```python
from build123d import *

# Parameters (mm, degrees)
BOSS_EXTRUDE1_DEPTH = 43.5102
CUT_EXTRUDE1_DEPTH  = 43.5102


with BuildPart() as part:
    # Sketch2 → Boss-Extrude1 (new body)
    with BuildSketch(Plane.XY):
        with BuildLine():
            Line((-4.366026501, 25.941944541), (-1.27, 34.448207442))
            ThreePointArc((-1.27, 34.448207442), (0, 34.47161), (1.27, 34.448207442))
            Line((1.27, 34.448207442), (4.366026501, 25.941944541))
            ThreePointArc((4.366026501, 25.941944541), (4.83385814, 25.858857079), (5.300112805, 25.767333549))
            Line((5.300112805, 25.767333549), (11.259888122, 32.580773709))
            ThreePointArc((11.259888122, 32.580773709), (12.452581833, 32.143819028), (13.628367585, 31.663219877))
            Line((13.628367585, 31.663219877), (13.442509735, 22.612952173))
            ThreePointArc((13.442509735, 22.612952173), (13.848735094, 22.366475142), (14.250442508, 22.11270138))
            Line((14.250442508, 22.11270138), (22.26906596, 26.31312595))
            ThreePointArc((22.26906596, 26.31312595), (23.223373486, 25.474827181), (24.14614861, 24.601939015))
            Line((24.14614861, 24.601939015), (20.703507542, 16.229955312))
            ThreePointArc((20.703507542, 16.229955312), (20.993263634, 15.8533768), (21.276170986, 15.471626358))
            Line((21.276170986, 15.471626358), (30.270683044, 16.491744725))
            ThreePointArc((30.270683044, 16.491744725), (30.857719866, 15.365318762), (31.402858467, 14.218029965))
            Line((31.402858467, 14.218029965), (25.168381933, 7.655013053))
            ThreePointArc((25.168381933, 7.655013053), (25.302535593, 7.199192074), (25.428434676, 6.741022466))
            Line((25.428434676, 6.741022466), (34.184076646, 4.443061991))
            ThreePointArc((34.184076646, 4.443061991), (34.324560189, 3.180638903), (34.418438279, 1.913897183))
            Line((34.418438279, 1.913897183), (26.234126882, -1.953781138))
            ThreePointArc((26.234126882, -1.953781138), (26.194559914, -2.427283433), (26.14644736, -2.899993864))
            Line((26.14644736, -2.899993864), (33.480721277, -8.205680884))
            ThreePointArc((33.480721277, -8.205680884), (33.155678459, -9.433603865), (32.785617282, -10.648718018))
            Line((32.785617282, -10.648718018), (23.756807626, -11.298706359))
            ThreePointArc((23.756807626, -11.298706359), (23.54886377, -11.725940863), (23.333237446, -12.149349953))
            Line((23.333237446, -12.149349953), (28.255608976, -19.746201087))
            ThreePointArc((28.255608976, -19.746201087), (27.508938632, -20.773786158), (26.724917, -21.773164845))
            Line((26.724917, -21.773164845), (18.07099986, -19.117678678))
            ThreePointArc((18.07099986, -19.117678678), (17.722763084, -19.440945003), (17.36874452, -19.757869009))
            Line((17.36874452, -19.757869009), (19.214420114, -28.619887416))
            ThreePointArc((19.214420114, -28.619887416), (18.14696421, -29.308353518), (17.054868589, -29.95702511))
            Line((17.054868589, -29.95702511), (9.944603428, -24.354702557))
            ThreePointArc((9.944603428, -24.354702557), (9.503105039, -24.530341795), (9.058506404, -24.697978373))
            Line((9.058506404, -24.697978373), (7.578217344, -33.628299361))
            ThreePointArc((7.578217344, -33.628299361), (6.334141716, -33.884665333), (5.081465671, -34.095023136))
            Line((5.081465671, -34.095023136), (0.475133198, -26.302488901))
            ThreePointArc((0.475133198, -26.302488901), (0, -26.30678), (-0.475133198, -26.302488901))
            Line((-0.475133198, -26.302488901), (-5.081465671, -34.095023136))
            ThreePointArc((-5.081465671, -34.095023136), (-6.334141716, -33.884665333), (-7.578217344, -33.628299361))
            Line((-7.578217344, -33.628299361), (-9.058506404, -24.697978373))
            ThreePointArc((-9.058506404, -24.697978373), (-9.503105039, -24.530341795), (-9.944603428, -24.354702557))
            Line((-9.944603428, -24.354702557), (-17.054868589, -29.95702511))
            ThreePointArc((-17.054868589, -29.95702511), (-18.14696421, -29.308353518), (-19.214420114, -28.619887416))
            Line((-19.214420114, -28.619887416), (-17.36874452, -19.757869009))
            ThreePointArc((-17.36874452, -19.757869009), (-17.722763084, -19.440945003), (-18.07099986, -19.117678678))
            Line((-18.07099986, -19.117678678), (-26.724917, -21.773164845))
            ThreePointArc((-26.724917, -21.773164845), (-27.508938632, -20.773786158), (-28.255608976, -19.746201087))
            Line((-28.255608976, -19.746201087), (-23.333237446, -12.149349953))
            ThreePointArc((-23.333237446, -12.149349953), (-23.54886377, -11.725940863), (-23.756807626, -11.298706359))
            Line((-23.756807626, -11.298706359), (-32.785617282, -10.648718018))
            ThreePointArc((-32.785617282, -10.648718018), (-33.155678459, -9.433603865), (-33.480721277, -8.205680884))
            Line((-33.480721277, -8.205680884), (-26.14644736, -2.899993864))
            ThreePointArc((-26.14644736, -2.899993864), (-26.194559914, -2.427283433), (-26.234126882, -1.953781138))
            Line((-26.234126882, -1.953781138), (-34.418438279, 1.913897183))
            ThreePointArc((-34.418438279, 1.913897183), (-34.324560189, 3.180638903), (-34.184076646, 4.443061991))
            Line((-34.184076646, 4.443061991), (-25.428434676, 6.741022466))
            ThreePointArc((-25.428434676, 6.741022466), (-25.302535593, 7.199192074), (-25.168381933, 7.655013053))
            Line((-25.168381933, 7.655013053), (-31.402858467, 14.218029965))
            ThreePointArc((-31.402858467, 14.218029965), (-30.857719866, 15.365318762), (-30.270683044, 16.491744725))
            Line((-30.270683044, 16.491744725), (-21.276170986, 15.471626358))
            ThreePointArc((-21.276170986, 15.471626358), (-20.993263634, 15.8533768), (-20.703507542, 16.229955312))
            Line((-20.703507542, 16.229955312), (-24.14614861, 24.601939015))
            ThreePointArc((-24.14614861, 24.601939015), (-23.223373486, 25.474827181), (-22.26906596, 26.31312595))
            Line((-22.26906596, 26.31312595), (-14.250442508, 22.11270138))
            ThreePointArc((-14.250442508, 22.11270138), (-13.848735094, 22.366475142), (-13.442509735, 22.612952173))
            Line((-13.442509735, 22.612952173), (-13.628367585, 31.663219877))
            ThreePointArc((-13.628367585, 31.663219877), (-12.452581833, 32.143819028), (-11.259888122, 32.580773709))
            Line((-11.259888122, 32.580773709), (-5.300112805, 25.767333549))
            ThreePointArc((-5.300112805, 25.767333549), (-4.83385814, 25.858857079), (-4.366026501, 25.941944541))
        make_face()
    extrude(amount=BOSS_EXTRUDE1_DEPTH)

    # Sketch4 → Cut-Extrude1 (cut)
    with BuildSketch(Plane.XY.offset(43.5102)):
        with BuildLine():
            Line((-3.175, 25.4), (3.175, 25.4))
            Line((3.175, 25.4), (3.175, 21.997045256))
            ThreePointArc((3.175, 21.997045256), (0, -22.225), (-3.175, 21.997045256))
            Line((-3.175, 21.997045256), (-3.175, 25.4))
        make_face()
    extrude(amount=-CUT_EXTRUDE1_DEPTH, mode=Mode.SUBTRACT)


solid = part.part
```
Geometry: final body of the model. Coordinates: model frame, mm. A direction names the side the tool comes from. Round coordinates to 2 decimals unless told otherwise and drop trailing zeros. Order: outer loops, then holes, each group sorted by start corner. A loop starts at its lowest first (then second) coordinate and runs counter-clockwise, first axis right, second up. Notation, with made-up numbers: M 32,61.5 L 46,61.5 A26 ccw 46,83.5 Z; hole C 44,40.5 d7. An arc over 180 degrees is marked long. One line per item, written item: value.
(1) Cut plane A-A (y = 0). Return the cut outline in (x, z) (3 decimals).
Result sheet:
outline: M -30.368,0 L -22.225,0 L -22.225,43.51 L -30.368,43.51 Z; M 22.225,0 L 30.368,0 L 30.368,43.51 L 22.225,43.51 Z
(2) Reachability of faces 1 (the flat face through (-8.308, -29.226, 21.451)), 2 (the flat face through (0, 25.4, 22)), 3 (the flat face through (25.76, -15.895, 21.451)) from +Z, -Z, +X, -X, +Y, -Y: full face, straight path, thin tool, end or side. Return the list, or none.
Result sheet:
face 1: +Z, -Z, -Y
face 2: +Z, -Z
face 3: +Z, -Z, +X
(3) Pin query (flat end, axial travel): P1, Ø1, axis at x = 12, y = -18.5, coming from the +Z side; P2, Ø8, axis at y = 11.5, z = 29, coming from the +X side; P3, Ø8, axis at x = -25, z = 28, coming from the +Y side; P4, Ø2.5, axis at y = 23.5, z = 29.5, coming from the +X side. Return the tip coordinate at first contact, or that it passes through.
Result sheet:
P1: z = 43.51
P2: x = 31.4
P3: y = 26.31
P4: x = 24.15
(4) Line query: probe 1 along Y at (x, z) = (0, 14) (3 decimals); probe 2 along X at (y, z) = (-29, 12); probe 3 along X at (y, z) = (26, 24). Output: solid intervals per line, ascending. Write a range as [from, to].
Result sheet:
probe 1: [-26.307, -22.225], [25.4, 34.472]
probe 2: [-18.64, -15.84], [-8.35, -2.07], [2.07, 8.35], [15.84, 18.64]
probe 3: [-22.63, -21.67], [-13.51, -5.5], [-4.34, 4.34], [5.5, 13.51], [21.67, 22.63]
(5) Cut plane B-B (y = 9.5). Return the cut outline in (x, z), and give its area (3 significant figures).
Result sheet:
outline: M -26.92,0 L -20.09,0 L -20.09,43.51 L -26.92,43.51 Z; M 20.09,0 L 26.92,0 L 26.92,43.51 L 20.09,43.51 Z
area: 594 mm2
(6) Pull-direction query (Y, two-part tool) for faces 4 (the cylindrical face through (-12.469, 32.137, 21.451)), 5 (the flat face through (25.71, 15.975, 21.451)), 6 (the flat face through (-2.746, -30.144, 21.451)); classes: pulls with the +Y half, pulls with the -Y half, needs draft (parallel to the pull), parting line crosses it, or undercut.
Result sheet:
face 4: pulls with the +Y half
face 5: undercut
face 6: pulls with the -Y half
